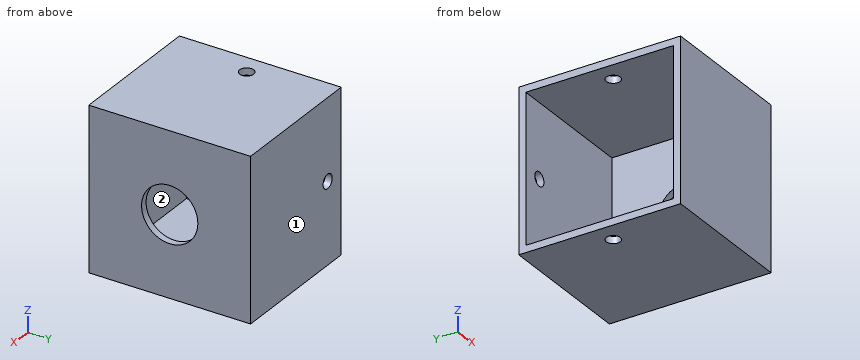
from build123d import *

# Parameters (mm, degrees)
F0_W     = 58.42
F0_H     = 58.42
F1_DEPTH = 50.8
F2_T     = -2.54
F3_R     = 10.16
F4_DEPTH = 25.4
F5_R     = 2.54
F6_DEPTH = 39.116
F7_R     = 2.54
F8_DEPTH = 80.01


with BuildPart() as f1:
    # F0 (on Right) → F1 (new body)
    with BuildSketch(Plane.YZ):
        Rectangle(F0_W, F0_H)
    extrude(amount=F1_DEPTH)

    # F2
    f2_openings = [f1.faces().sort_by_distance(p)[0] for p in [
        (0, 0, 0),
    ]]
    offset(amount=F2_T, openings=f2_openings)

    # F3 (on face) → F4 (cut)
    with BuildSketch(Plane.YZ.offset(50.8)):
        Circle(F3_R)
    extrude(amount=-F4_DEPTH, mode=Mode.SUBTRACT)

    # F5 (on face) → F6 (cut)
    with BuildSketch(Plane(origin=(0, 29.21, 0), x_dir=(-1, 0, 0), z_dir=(0, 1, 0))):
        with Locations((-7.62, 0)):
            Circle(F5_R)
    extrude(amount=-F6_DEPTH, mode=Mode.SUBTRACT)

    # F7 (on face) → F8 (cut)
    with BuildSketch(Plane(origin=(0, 0, -29.21), x_dir=(1, 0, 0), z_dir=(0, 0, -1))):
        with Locations((7.62, 0)):
            Circle(F7_R)
    extrude(amount=-F8_DEPTH, mode=Mode.SUBTRACT)


solid = f1.part
Design review of the part built by this model. Coordinates are the model's own, in mm. Face numbers are marked on the shaded views. A direction names the side the tool comes from. Coordinates: 2 decimals unless noted, no trailing zeros. Loops run counter-clockwise (first coordinate to the right, second up) from the corner with the lowest first, then second, coordinate; pieces in that order, holes last. Notation, with made-up numbers: M 63.5,-12.75 L 72.5,-12.75 A19 ccw 72.5,16.25 Z; hole C 27,14 d5. An arc over 180 degrees is marked long. Use one line per item in the form item = value.
(1) For the marked faces 1 and 2, list the 3-axis set-ups (+Z, -Z, +X, -X, +Y, -Y) from which the entire face can be reached by the end or side of a thin tool; tool diameter is ignored.
Return value:
face_1 = +Z, -Z, +X, -X, +Y
face_2 = -X
(2) Consider section B-B (z = 0). Write out the cut boundary in (x, y), and give its area (3 significant figures).
Return value:
outline = M 0,-29.21 L 50.8,-29.21 L 50.8,-10.16 L 48.26,-10.16 L 48.26,-26.67 L 0,-26.67 Z; M 0,26.67 L 5.08,26.67 L 5.08,29.21 L 0,29.21 Z; M 10.16,26.67 L 48.26,26.67 L 48.26,10.16 L 50.8,10.16 L 50.8,29.21 L 10.16,29.21 Z
area = 329 mm2
(3) For line 1 along Z through (x, y) = (49, 0); line 2 along Y through (x, z) = (35, 25), list the stretches that pass through material, from the lowest coordinate up. Write a range as from..to.
Return value:
line_1 = -29.21..-10.16, 10.16..29.21
line_2 = -29.21..-26.67, 26.67..29.21
(4) Consider section C-C (x = 7.62). Write out the cut boundary in (y, z).
Return value:
outline = M -29.21,-29.21 L -2.54,-29.21 L -2.54,-26.67 L -26.67,-26.67 L -26.67,26.67 L -2.54,26.67 L -2.54,29.21 L -29.21,29.21 Z; M 2.54,-29.21 L 29.21,-29.21 L 29.21,-2.54 L 26.67,-2.54 L 26.67,-26.67 L 2.54,-26.67 Z; M 2.54,26.67 L 26.67,26.67 L 26.67,2.54 L 29.21,2.54 L 29.21,29.21 L 2.54,29.21 Z
(5) Consider section A-A (y = 0). Write out the cut boundary in (x, z).
Return value:
outline = M 0,-29.21 L 5.08,-29.21 L 5.08,-26.67 L 0,-26.67 Z; M 0,26.67 L 5.08,26.67 L 5.08,29.21 L 0,29.21 Z; M 10.16,-29.21 L 50.8,-29.21 L 50.8,-10.16 L 48.26,-10.16 L 48.26,-26.67 L 10.16,-26.67 Z; M 10.16,26.67 L 48.26,26.67 L 48.26,10.16 L 50.8,10.16 L 50.8,29.21 L 10.16,29.21 Z
(6) Consider section D-D (x = 36). Write out the cut boundary in (y, z).
Return value:
outline = M -29.21,-29.21 L 29.21,-29.21 L 29.21,29.21 L -29.21,29.21 Z; hole M -26.67,-26.67 L 26.67,-26.67 L 26.67,26.67 L -26.67,26.67 Z
(7) Clearance check with flat-ended pins moving along their axes: P1, Ø6.5, axis at x = 7.62, y = 0, coming from the -Z side; P2, Ø12, axis at y = -20.5, z = -17.5, coming from the -X side; P3, Ø4.5, axis at x = 7.62, z = 0, coming from the +Y side. State where each tip first meets the part, or that it passes through.
Return value:
P1 = -29.21
P2 = 48.26
P3 = -26.67
